Check sheet for the modelled part. Datum: model origin and axes. Units: mm. A direction names the side the tool comes from. Round coordinates to 2 decimals unless told otherwise and drop trailing zeros. Order: outer loops, then holes, each group sorted by start corner. A loop starts at its lowest first (then second) coordinate and runs counter-clockwise, first axis right, second up. Notation, with made-up numbers: (71, 11) -> (95, 11) arc R16 ccw to (95, 16) -> close; hole circle Ø1 at (24, 60). An arc over 180 degrees is marked (long way). Answer in a Markdown table with one row per item.
from build123d import *

# Parameters (mm, degrees)
ESQUISSE1_W                  = 300
ESQUISSE1_H                  = 150
BOSS_EXTRU_1_DEPTH           = 5
ESQUISSE2_OUTSIDE_W          = 369.112
ESQUISSE2_OUTSIDE_H          = 219.112
ENL_V_MAT_EXTRU_1_DEPTH      = 5
ENL_V_MAT_EXTRU_2_DEPTH      = 336.559234711
ENL_V_MAT_EXTRU_2_DEPTH_BACK = 336.559234711
ENL_V_MAT_EXTRU_4_DEPTH      = 336.559234711
ENL_V_MAT_EXTRU_4_DEPTH_BACK = 336.559234711
ESQUISSE5_R                  = 3
ENL_V_MAT_EXTRU_5_DEPTH      = 49
EMPREINTE1_START             = -5
EMPREINTE1_DEPTH             = 10
D_PLACER_START               = -5
D_PLACER_LA_FACE1_DEPTH      = 10


# Read off the part's stored shape, not the designer's step: Empreinte1, Déplacer la face1
with BuildPart() as part:
    # Esquisse1 → Boss.-Extru.1 (new, symmetric)
    with BuildSketch(Plane(origin=(0, 0, 0), x_dir=(0, 0, -1), z_dir=(1, 0, 0))):
        with Locations((150, 75)):
            Rectangle(ESQUISSE1_W, ESQUISSE1_H)
    extrude(amount=BOSS_EXTRU_1_DEPTH, both=True)

    # Esquisse2 outside → Enlèv. mat.-Extru.1 (cut, symmetric)
    with BuildSketch(Plane(origin=(0, 0, 0), x_dir=(0, 0, -1), z_dir=(1, 0, 0))):
        with Locations((150, 75)):
            Rectangle(ESQUISSE2_OUTSIDE_W, ESQUISSE2_OUTSIDE_H)
        Polygon((0, 117.225703003), (60, 139.063917059), (185, 150), (300, 129.722397219), (300, 99.722397219), (211.741963761, 84.160124165), (171.741963761, 14.878091862), (139.835792798, 0), (29.835792798, 0), (0, 17.225703003), align=None, mode=Mode.SUBTRACT)
    extrude(amount=ENL_V_MAT_EXTRU_1_DEPTH, both=True, mode=Mode.SUBTRACT)

    # Esquisse3 → Enlèv. mat.-Extru.2 (cut, two sides: drawn at the far end of the back side and taken through both)
    with BuildSketch(Plane(origin=(5, 0, 0), x_dir=(0, 0, -1), z_dir=(1, 0, 0)).offset(-ENL_V_MAT_EXTRU_2_DEPTH_BACK)):
        Polygon((20, 103.221552239), (20, 80.493304508), (55, 74.321860183), (80, 88.755616913), (62.679491924, 118.755616913), align=None)
        Polygon((90, 71.435108837), (113.922571241, 30), (81.508057782, 49.831775443), align=None)
        Polygon((82.886751346, 123.755616913), (139.903333355, 25), (175.32640016, 86.354551467), (150.32640016, 129.655821657), align=None)
        Polygon((91.944969354, 20), (30, 20), (30, 48.267236345), (52.117107943, 44.367393479), align=None)
    extrude(amount=ENL_V_MAT_EXTRU_2_DEPTH + ENL_V_MAT_EXTRU_2_DEPTH_BACK, mode=Mode.SUBTRACT)

    # Esquisse5 → Enlèv. mat.-Extru.4 (cut, two sides: drawn at the far end of the back side and taken through both)
    with BuildSketch(Plane.ZY.offset(5).offset(-ENL_V_MAT_EXTRU_4_DEPTH_BACK)):
        with Locations((-275, 107.010571736)):
            Circle(ESQUISSE5_R)
    extrude(amount=ENL_V_MAT_EXTRU_4_DEPTH + ENL_V_MAT_EXTRU_4_DEPTH_BACK, mode=Mode.SUBTRACT)

    # Esquisse6 → Enlèv. mat.-Extru.5 (cut)
    with BuildSketch(Plane(origin=(5, 0, 0), x_dir=(0, 0, -1), z_dir=(1, 0, 0))):
        Polygon((205.171612033, 138.776729635), (224.867767093, 135.303766081), (223.825878027, 129.394919563), (204.129722967, 132.867883116), align=None)
    extrude(amount=-ENL_V_MAT_EXTRU_5_DEPTH, mode=Mode.SUBTRACT)

    # Empreinte1 outline → Empreinte1 (cut)
    with BuildSketch(Plane.YZ.offset(EMPREINTE1_START)):
        Polygon((97.361325712, 0), (93.361325712, 0), (91.051924635, -4), (99.670726788, -4), align=None)
        Polygon((35.051924635, -4), (43.670726788, -4), (41.361325712, 0), (37.361325712, 0), align=None)
    extrude(amount=EMPREINTE1_DEPTH, mode=Mode.SUBTRACT)

    # Déplacer la face1 outline → Déplacer la face1 (cut)
    with BuildSketch(Plane.YZ.offset(D_PLACER_START)):
        Polygon((93.361325712, 0), (93.072650577, 0), (90.618911933, -4.25), (100.10373949, -4.25), (97.650000846, 0), (97.361325712, 0), (99.670726788, -4), (91.051924635, -4), align=None)
        Polygon((34.618911933, -4.25), (44.10373949, -4.25), (41.650000846, 0), (41.361325712, 0), (43.670726788, -4), (35.051924635, -4), (37.361325712, 0), (37.072650577, 0), align=None)
    extrude(amount=D_PLACER_LA_FACE1_DEPTH, mode=Mode.SUBTRACT)


solid = part.part
Item 1: Cross-section at B-B (z = -275). Record the boundary of the cut face in (x, y).
Result sheet:
| item | result |
|---|---|
| outline | (-5, 95.31) -> (5, 95.31) -> (5, 104.01) -> (-5, 104.01) -> close; (-5, 110.01) -> (5, 110.01) -> (5, 134.13) -> (-5, 134.13) -> close |
Item 2: Cross-section at A-A (y = 65.5). Record the boundary of the cut face in (x, z).
Result sheet:
| item | result |
|---|---|
| outline | (-5, -200.97) -> (5, -200.97) -> (5, -163.29) -> (-5, -163.29) -> close; (-5, -116.52) -> (5, -116.52) -> (5, -93.43) -> (-5, -93.43) -> close; (-5, -87.67) -> (5, -87.67) -> (5, 0) -> (-5, 0) -> close |
Item 3: Mould release check, pull along Z, two halves, no side actions. Record for faces 1 (the flat face through (0, 107, 0)), 2 (the flat face through (0.07, 50, -192.02)), 3 (the flat face through (-0.1, 51, -101.8)): pulls with the +Z half, pulls with the -Z half, needs draft (parallel to the pull), parting line crosses it, or undercut.
Result sheet:
| item | result |
|---|---|
| face 1 | pulls with the +Z half |
| face 2 | pulls with the -Z half |
| face 3 | undercut |
Item 4: Set-up check for faces 4 (the flat face through (-0.07, 107.702, -163.001)), 5 (the flat face through (0, 67, 0)): record each of +Z, -Z, +X, -X, +Y, -Y from which the full face is reachable in a straight line by a thin tool's end or side.
Result sheet:
| item | result |
|---|---|
| face 4 | +X, -X |
| face 5 | +Z, +X, -X, +Y, -Y |
Item 5: Cross-section at D-D (y = 11). Record the boundary of the cut face in (x, z), and give its area (3 significant figures).
Result sheet:
| item | result |
|---|---|
| outline | (-5, -163.43) -> (5, -163.43) -> (5, -10.78) -> (-5, -10.78) -> close |
| area | 1,530 mm^2 |
Item 6: Scan lines: line 1 (Y direction, x = 4.25, z = -71); line 2 (Z direction, x = -3.5, y = 66); line 3 (Z direction, x = 3.5, y = 81). Record each from-to range of solid material in increasing order. Write a range as [from, to].
Result sheet:
| item | result |
|---|---|
| line 1 | y = [0, 20], [32.81, 83.56], [104.34, 140.03] |
| line 2 | z = [-201.26, -163.57], [-116.23, -93.14], [-87.86, 0] |
| line 3 | z = [-209.92, -172.23], [-107.57, -66.57], [-20, 0] |
Item 7: Cross-section at C-C (x = -1.25). State how many separate pieces and enclosed holes the cut face has, and give its area (3 significant figures).
Result sheet:
| item | result |
|---|---|
| separate pieces | 1 |
| enclosed holes | 6 |
| area | 22,700 mm^2 |
Item 8: Depth check by flat-ended pin: P1, Ø1, axis at x = -1.5, y = 26.5, coming from the -Z side; P2, Ø2, axis at x = 0, z = -80.5, coming from the -Y side; P3, Ø2, axis at x = 0, z = -100.5, coming from the +Y side; P4, Ø5, axis at x = 1, y = 25, coming from the -Z side. Enter the tip coordinate at first touch or a pass-through.
Result sheet:
| item | result |
|---|---|
| P1 | stops at z = -178.74 |
| P2 | stops at y = 0 |
| P3 | stops at y = 142.69 |
| P4 | stops at z = -179.03 |
